Here's how the part is built. I have some questions about the finished solid (model axes, mm). A direction names the side the tool comes from. Coordinates: 2 decimals unless noted, no trailing zeros. Write each loop counter-clockwise with the first axis right and the second up, starting at its lowest first coordinate (ties: lowest second). Pieces come first, ordered by that corner, then holes. Notation, with made-up numbers: (86, -35.5) -> (127, -35.5) arc R13 ccw to (127, -12.5) -> close; hole circle Ø4 at (16.5, 56). An arc over 180 degrees is marked (long way). Use a Markdown table: item, result. Add a question column.
```python
from build123d import *

# Parameters (mm, degrees)
SKETCH_1_W          = 36
SKETCH_1_H          = 24
EXTRUDE_1_DEPTH     = 50
SKETCH_2_R          = 4.5
CUT_EXTRUDE_1_DEPTH = 36
SKETCH_3_R          = 3.4
CUT_EXTRUDE_2_DEPTH = 6
SKETCH_5_W          = 18
SKETCH_5_H          = 10
EXTRUDE_2_DEPTH     = 36
SKETCH_6_R          = 1.6
CUT_EXTRUDE_3_DEPTH = 5


with BuildPart() as part:
    # 草图1 → 凸台-拉伸1 (new body)
    with BuildSketch(Plane(origin=(0, 0, 0), x_dir=(1, 0, 0), z_dir=(0, 1, 0))):
        with Locations((18, 12)):
            Rectangle(SKETCH_1_W, SKETCH_1_H)
    extrude(amount=EXTRUDE_1_DEPTH)

    # 草图2 → 切除-拉伸1 (cut)
    with BuildSketch(Plane.ZY):
        with Locations((-14, 20)):
            Circle(SKETCH_2_R)
    extrude(amount=-CUT_EXTRUDE_1_DEPTH, mode=Mode.SUBTRACT)

    # 草图3 → 切除-拉伸2 (cut)
    with BuildSketch(Plane.XY):
        with Locations((8, 10)):
            Circle(SKETCH_3_R)
        with Locations((28, 10)):
            Circle(SKETCH_3_R)
    extrude(amount=-CUT_EXTRUDE_2_DEPTH, mode=Mode.SUBTRACT)

    # 草图5 → 凸台-拉伸2 (add)
    with BuildSketch(Plane(origin=(36, 0, 0), x_dir=(0, 0, -1), z_dir=(1, 0, 0))):
        with Locations((-9, 45)):
            Rectangle(SKETCH_5_W, SKETCH_5_H)
    extrude(amount=-EXTRUDE_2_DEPTH)

    # 草图6 → 切除-拉伸3 (cut)
    with BuildSketch(Plane(origin=(0, 50, 0), x_dir=(1, 0, 0), z_dir=(0, 1, 0))):
        with Locations(Location((26, -12.5, 0), (0, 0, 270))):
            Circle(SKETCH_6_R)
        with Locations(Location((10, -12.5, 0), (0, 0, 270))):
            Circle(SKETCH_6_R)
    extrude(amount=-CUT_EXTRUDE_3_DEPTH, mode=Mode.SUBTRACT)


solid = part.part
```
Q1. Suppose I cut it at A-A, the plane z = -14. Write out the boundary of the cut face in (x, y).
Q2. Please list where these lines run through material, in increasing order: line 1 (Y direction, x = 28, z = -4.2); line 2 (X direction, y = 48, z = 12); line 3 (Y direction, x = 27.5, z = -14).
Q3. Thinking about a two-plate mould opening in Z: for faces 5 (the flat face through (36, 31, -7)), 6 (the flat face through (18, 45, 18)), 7 (the cylindrical face through (10.07, 47.54, 10.9)), which applies, released by +Z, released by -Z, zero draft, split by the parting line, or undercut?
Q4. Suppose I cut it at D-D, the plane y = 10. Write out the boundary of the cut face in (x, z).
Q5. Suppose I cut it at C-C, the plane x = 32. Write out the boundary of the cut face in (y, z).
Q6. Suppose I cut it at B-B, the plane y = 20. Write out the boundary of the cut face in (x, z), and give its area (3 significant figures).
Q7. Which directions (+Z, -Z, +X, -X, +Y, -Y) give clear straight access to the entire face, cutting with the end or side of a thin tool? Please do faces 1 (the cylindrical face through (29.6, 7, -3)), 2 (the flat face through (10, 45, 12)), 3 (the flat face through (18, 0, -12)), 4 (the flat face through (18, 20, 0)).
Q8. Will these pins go through, and if not, where does the flat tip stop? pin 1 (1 mm diameter, centred on x = 29, y = 18, fed in from +Z); pin 2 (4 mm diameter, centred on x = 28, y = 10, fed in from +Z); pin 3 (1 mm diameter, centred on x = 26.5, z = 13, fed in from +Y).
Answer key:
| question | item | result |
|---|---|---|
| 1 | outline | (0, 0) -> (36, 0) -> (36, 15.5) -> (0, 15.5) -> close; (0, 24.5) -> (36, 24.5) -> (36, 50) -> (0, 50) -> close |
| 2 | line 1 | y = 0 to 6.6, 13.4 to 50 |
| 2 | line 2 | x = 0 to 8.48, 11.52 to 24.48, 27.52 to 36 |
| 2 | line 3 | y = 0 to 15.5, 24.5 to 50 |
| 3 | face 5 | zero draft |
| 3 | face 6 | released by +Z |
| 3 | face 7 | undercut |
| 4 | outline | (0, -24) -> (36, -24) -> (36, 0) -> (31.4, 0) -> (31.4, -6) -> (24.6, -6) -> (24.6, 0) -> (11.4, 0) -> (11.4, -6) -> (4.6, -6) -> (4.6, 0) -> (0, 0) -> close |
| 5 | outline | (0, -24) -> (50, -24) -> (50, 18) -> (40, 18) -> (40, 0) -> (0, 0) -> close; hole circle Ø9 at (20, -14) |
| 6 | outline | (0, -24) -> (36, -24) -> (36, -18.5) -> (0, -18.5) -> close; (0, -9.5) -> (36, -9.5) -> (36, 0) -> (0, 0) -> close |
| 6 | area | 540 mm^2 |
| 7 | face 1 | +Z |
| 7 | face 2 | +Y |
| 7 | face 3 | +Z, -Z, +X, -X, -Y |
| 7 | face 4 | +Z, +X, -X, -Y |
| 8 | pin 1 | stops at z = 0 |
| 8 | pin 2 | stops at z = -6 |
| 8 | pin 3 | stops at y = 45 |
